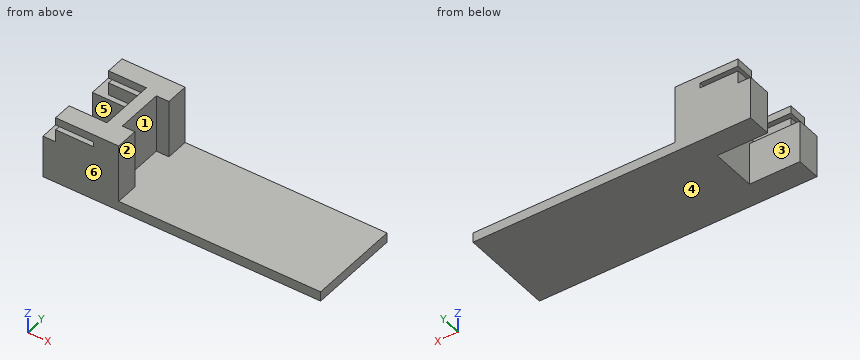
from build123d import *

# Parameters (mm, degrees)
F1_DEPTH  = 37
F2_W      = 19
F2_H      = 23.015723977
F3_DEPTH  = 5
F4_W      = 18
F4_H      = 26.8701749424
F5_DEPTH  = 20
F6_W      = 37
F6_H      = 2
F7_DEPTH  = 20
F8_W      = 37
F8_H      = 10
F9_DEPTH  = 5
F10_W     = 20
F10_H     = 22
F11_DEPTH = 10


with BuildPart() as f1:
    # F0 (on Front) → F1 (new body)
    with BuildSketch(Plane.XZ):
        Polygon((15.5247052472, -27.7605104941), (-14.4752947528, -27.7605104941), (-14.4752947528, -54.6306854365), (15.5247052472, -54.6306854365), (95.5247052472, -54.6306854365), (95.5247052472, -50.776234471), (15.5247052472, -50.776234471), align=None)
    extrude(amount=F1_DEPTH)

    # F2 (on face) → F3 (cut)
    with BuildSketch(Plane.YZ.offset(15.5247052472)):
        with Locations((-18.5, -39.2683724826)):
            Rectangle(F2_W, F2_H)
    extrude(amount=-F3_DEPTH, mode=Mode.SUBTRACT)

    # F4 (on face) → F5 (cut)
    with BuildSketch(Plane(origin=(-14.4752947528, 0, 0), x_dir=(0, -1, 0), z_dir=(-1, 0, 0))):
        with Locations((18.5, -41.1955979653)):
            Rectangle(F4_W, F4_H)
    extrude(amount=-F5_DEPTH, mode=Mode.SUBTRACT)

    # F6 (on face) → F7 (cut, through all)
    with BuildSketch(Plane(origin=(-14.4752947528, 0, 0), x_dir=(0, -1, 0), z_dir=(-1, 0, 0))):
        with Locations((18.5, -31.7605104941)):
            Rectangle(F6_W, F6_H)
    extrude(amount=-F7_DEPTH, mode=Mode.SUBTRACT)

    # F8 (on face) → F9 (cut)
    with BuildSketch(Plane(origin=(-14.4752947528, 0, 0), x_dir=(0, -1, 0), z_dir=(-1, 0, 0))):
        with Locations((18.5, -32.7605104941)):
            Rectangle(F8_W, F8_H)
    extrude(amount=-F9_DEPTH, mode=Mode.SUBTRACT)

    # F10 (on face) → F11 (cut, through all)
    with BuildSketch(Plane.XY.offset(-27.7605104941)):
        with Locations((-4.4752947528, -18.5)):
            Rectangle(F10_W, F10_H)
    extrude(amount=-F11_DEPTH, mode=Mode.SUBTRACT)


solid = f1.part
Design review of the part built by this model. Coordinates are the model's own, in mm. Face numbers are marked on the shaded views. A direction names the side the tool comes from. Give positions to 0.01 mm unless a question says otherwise; leave off trailing zeros. Loops run counter-clockwise (first coordinate to the right, second up) from the corner with the lowest first, then second, coordinate; pieces in that order, holes last. Notation, with made-up numbers: (37, 17.5) - (79, 17.5) arc R26 cw to (79, 43.5) - close; hole circle Ø2 at (72, 32.5). An arc over 180 degrees is marked (long way). Use CSV: the item, a comma, the result in double quotes. Start each with the question number.
1. Add section A-A (x = -7). State the section outline as (y, z) points, plus the area to 3 significant figures.
2. Add section B-B (y = -5.5). State the section outline as (x, z) points.
3. Machinability: for the marked faces 1, 2 and 3, which of the approach directions +Z, -Z, +X, -X, +Y, -Y give a long, thin tool a straight path to every point of the face, cutting with its end or side? Answer none if there is none.
4. Insertion check: P1, Ø7, axis at y = -34, z = -38.5, coming from the +X side; P2, Ø1.5, axis at y = -26.5, z = -35.5, coming from the +X side; P3, Ø1.5, axis at y = -3, z = -35.5, coming from the -X side; P4, Ø10, axis at x = 78, z = -41, coming from the +Y side. Each pin has a flat end and moves straight along its axis. Give the tip position at first contact, or say it passes through.
5. Add section C-C (z = -34.75). State the section outline as (x, y) points, plus the area to 3 significant figures.
6. Add section D-D (y = -17.5). State the section outline as (x, z) points, plus the area to 3 significant figures.
7. Draft analysis for pull direction Y (two halves, no side actions). For the marked faces 4, 5 and 6, state which applies: released by +Y, released by -Y, zero draft, split by the parting line, or undercut.
8. Wall thickness on L1, parallel to Z at x = 3.5, y = -6.5; L2, parallel to X at y = -13.5, z = -35.5; L3, parallel to Y at x = -2.5, z = -29: over which ranges is each line inside the solid? List them lowest first.
Results found:
1,outline,"(-37, -54.63) - (-27.5, -54.63) - (-27.5, -37.76) - (-29.5, -37.76) - (-29.5, -32.76) - (-37, -32.76) - close; (-37, -30.76) - (-29.5, -30.76) - (-29.5, -27.76) - (-37, -27.76) - close; (-9.5, -54.63) - (0, -54.63) - (0, -32.76) - (-7.5, -32.76) - (-7.5, -37.76) - (-9.5, -37.76) - close; (-7.5, -30.76) - (0, -30.76) - (0, -27.76) - (-7.5, -27.76) - close"
1,area,"441 mm²"
2,outline,"(-14.48, -54.63) - (95.52, -54.63) - (95.52, -50.78) - (15.52, -50.78) - (15.52, -27.76) - (-9.48, -27.76) - (-9.48, -30.76) - (5.52, -30.76) - (5.52, -32.76) - (-9.48, -32.76) - (-9.48, -37.76) - (-14.48, -37.76) - close"
3,face 1,"+Z, +X"
3,face 2,"+Z, +X, +Y, -Y"
3,face 3,"+Z, -Z, -X"
4,P1,"stops at x = 15.52"
4,P2,"stops at x = 10.52"
4,P3,"stops at x = -9.48"
4,P4,"passes through"
5,outline,"(-9.48, -37) - (15.52, -37) - (15.52, -28) - (10.52, -28) - (10.52, -9) - (15.52, -9) - (15.52, 0) - (-9.48, 0) - (-9.48, -7.5) - (5.52, -7.5) - (5.52, -29.5) - (-9.48, -29.5) - close"
5,area,"500 mm²"
6,outline,"(5.52, -54.63) - (95.52, -54.63) - (95.52, -50.78) - (10.52, -50.78) - (10.52, -27.76) - (5.52, -27.76) - close"
6,area,"462 mm²"
7,face 4,"zero draft"
7,face 5,"undercut"
7,face 6,"released by -Y"
8,L1,"z = -54.63 to -32.76, -30.76 to -27.76"
8,L2,"x = 5.52 to 10.52"
8,L3,"y = -37 to -29.5, -7.5 to 0"
